Model file for the job. Use its own axes, mm. Face numbers are marked on the shaded views. A direction names the side the tool comes from. Round coordinates to 2 decimals unless told otherwise and drop trailing zeros. Loops run counter-clockwise (first coordinate to the right, second up) from the corner with the lowest first, then second, coordinate; pieces in that order, holes last. Notation, with made-up numbers: M 34,56 L 44,56 A22 cw 44,87 Z; hole C 31.5,54 d10. An arc over 180 degrees is marked long. Use a Markdown table: item, result. Add a question column.
Item 1: Pin check, flat tips, straight feed: P1, Ø1.5, axis at y = 10, z = 7, coming from the +X side; P2, Ø0.6, axis at y = 14, z = 4.5, coming from the +X side; P3, Ø1.8, axis at y = 13.5, z = 3.5, coming from the -X side. Stop position of each tip, or through.
Item 2: Two-plate mould, pull along X, no slides. Class the marked faces 4, 5, 6 and 7: +X half, -X half, draft (parallel to the pull), parting line (faces both ways), or undercut.
Item 3: Saw through at D-D on x = 0. Write the cut outline in (y, z), then the cut area to 3 significant figures.
Item 4: Tool access for the marked faces 1, 2 and 3: list every direction of +Z, -Z, +X, -X, +Y, -Y with a clear straight run to the whole face (end or side of a thin tool).
Item 5: Wall check: L1, parallel to X at y = 8, z = 4; L2, parallel to X at y = 13.75, z = 2.5; L3, parallel to Y at x = 0, z = 2.75. Give the ranges that are in metal, low to high. Write a range as from..to.
Item 6: Saw through at A-A on y = 12.25. Write the cut outline in (x, z), then the cut area to 3 significant figures.
Item 7: Saw through at B-B on x = -3.75. Write the cut outline in (y, z).
Autodesk Inventor part; units mm, degrees
ref_plane "YZ Plane" through (0, 0, 0) normal (1, 0, 0) x (0, 1, 0)
ref_plane "XZ Plane" through (0, 0, 0) normal (0, 1, 0) x (-1, 0, 0)
ref_plane "XY Plane" through (0, 0, 0) normal (0, 0, 1) x (1, 0, 0)
sketch "Sketch3" plane through (0, 0, 0) normal (0, 0, 1) x (1, 0, 0)
  line L0 (-6.25, 1) -> (-6.25, 8)
  line L1 (6.25, 1) -> (6.25, 8)
  arc A0 (-1.5, 12.7697) -> (1.5, 12.7697) centre (0, 8) ccw
  line L2 (-3, 13.4829) -> (-3, 16)
  line L3 (-3, 16) -> (-1.5, 16)
  line L4 (1.5, 16) -> (3, 16)
  line L5 (3, 16) -> (3, 13.4829)
  arc A1 (-3, 13.4829) -> (-6.25, 8) centre (0, 8) ccw
  arc A2 (6.25, 8) -> (3, 13.4829) centre (0, 8) ccw
  line L6 (6.25, 1) -> (-6.25, 1)
  line L7 (-1.5, 16) -> (-1.5, 12.7697)
  line L8 (1.5, 12.7697) -> (1.5, 16)
  point P0 (0, 0)
  dimension "d10" = 10
  dimension "d12" = 8
  dimension "d13" = 1.5
  dimension "d21" = 1.25
  dimension "d22" = 1.25
  dimension "d24" = 7
  dimension "d25" = 8
  dimension "d26" = 3
extrude "Extrusion1" add sketch "Sketch3" along normal blind 8
fillet "Fillet1" radius 1 2 edges at (-1.5, 16, 4) (1.5, 16, 4)
fillet "Fillet2" radius 0.5 2 edges at (3, 16, 4) (-3, 16, 4)
properties part number "WireClip10"
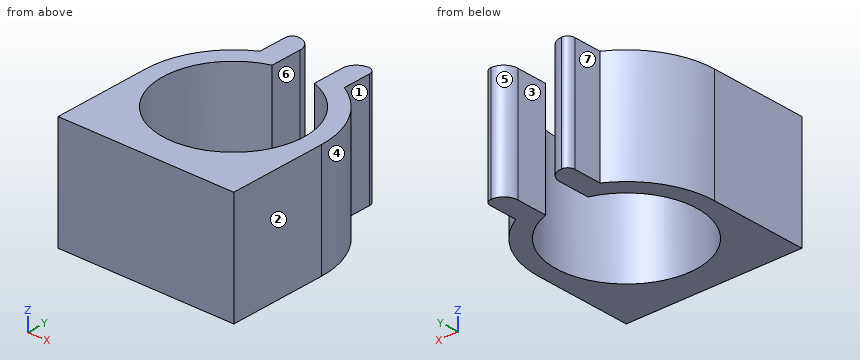
Entries:
| question | item | result |
|---|---|---|
| 1 | P1 | x = 6.12 |
| 1 | P2 | x = 3 |
| 1 | P3 | x = -4.23 |
| 2 | face 4 | +X half |
| 2 | face 5 | undercut |
| 2 | face 6 | undercut |
| 2 | face 7 | -X half |
| 3 | outline | M 1,0 L 3,0 L 3,8 L 1,8 Z |
| 3 | area | 16.0 mm2 |
| 4 | face 1 | +Z, -Z, +X, +Y |
| 4 | face 2 | +Z, -Z, +X, +Y, -Y |
| 4 | face 3 | +Z, -Z, +Y |
| 5 | L1 | -6.25..-5, 5..6.25 |
| 5 | L2 | -3..-1.5, 1.5..3 |
| 5 | L3 | 1..3 |
| 6 | outline | M -4.58,0 L -2.63,0 L -2.63,8 L -4.58,8 Z; M 2.63,0 L 4.58,0 L 4.58,8 L 2.63,8 Z |
| 6 | area | 31.2 mm2 |
| 7 | outline | M 1,0 L 4.69,0 L 4.69,8 L 1,8 Z; M 11.31,0 L 13,0 L 13,8 L 11.31,8 Z |
